from build123d import *

# Parameters (mm, degrees)
SKETCH2_R                                 = 1
SKETCH2_W                                 = 23
SKETCH2_H                                 = 12
BOSS_EXTRUDE1_DEPTH                       = 6
CUT_EXTRUDE1_REACH                        = 57.536
SKETCH3_W                                 = 10
SKETCH3_H                                 = 11
FILLET1_R                                 = 3
TAP_DRILL_FOR_M3X0_5_TAP1_D               = 2.5
TAP_DRILL_FOR_M3X0_5_TAP1_DEPTH           = 10
TAP_DRILL_FOR_M3X0_5_TAP1_TIP             = 0.751075774
TAP_DRILL_FOR_M3X0_5_TAP1_ON_FACE_2_D     = 2.5
TAP_DRILL_FOR_M3X0_5_TAP1_ON_FACE_2_DEPTH = 10
TAP_DRILL_FOR_M3X0_5_TAP1_ON_FACE_2_TIP   = 0.751075774


with BuildPart() as part:
    # Sketch2 → Boss-Extrude1 (new body)
    with BuildSketch(Plane(origin=(0, 0, 0), x_dir=(0, 0, -1), z_dir=(1, 0, 0))):
        Polygon((-20, 0), (-22.339658165, -13.268860813), (-43.5, -17), (-43.5, -34), (0, -34), (0, 0), align=None)
        with Locations(Location((-41.25, -25, 0), (0, 0, 180))):
            Circle(SKETCH2_R, mode=Mode.SUBTRACT)
        with Locations(Location((-13.75, -25, 0), (0, 0, 180))):
            Circle(SKETCH2_R, mode=Mode.SUBTRACT)
        with Locations((-27.5, -25)):
            Rectangle(SKETCH2_W, SKETCH2_H, mode=Mode.SUBTRACT)
    extrude(amount=BOSS_EXTRUDE1_DEPTH)

    # Sketch3 → Cut-Extrude1 (cut, up to next)
    with BuildSketch(Plane.ZY, mode=Mode.PRIVATE) as cut_extrude1_sk1:
        with Locations((5, -28.5)):
            Rectangle(SKETCH3_W, SKETCH3_H)
    cut_extrude1_tool1 = extrude(cut_extrude1_sk1.sketch, amount=-CUT_EXTRUDE1_REACH, mode=Mode.PRIVATE) & part.part
    add(cut_extrude1_tool1.solids().sort_by_distance((0, -28.5, 5))[0], mode=Mode.SUBTRACT)

    # Fillet1
    fillet1_edges = [part.edges().sort_by_distance(p)[0] for p in [
        (3, -34, 43.5),
        (3, -17, 43.5),
        (3, -13.268860813, 22.339658165),
        (3, -34, 10),
    ]]
    fillet(fillet1_edges, radius=FILLET1_R)

    # Tap Drill for M3x0.5 Tap1
    with Locations(Plane(origin=(3, 0, 3), x_dir=(0, 0, 1), z_dir=(0, 1, 0))):
        with Locations((0, 0), (14, 0)):
            Hole(TAP_DRILL_FOR_M3X0_5_TAP1_D / 2, depth=TAP_DRILL_FOR_M3X0_5_TAP1_DEPTH)
            with Locations((0, 0, -(TAP_DRILL_FOR_M3X0_5_TAP1_DEPTH + TAP_DRILL_FOR_M3X0_5_TAP1_TIP / 2))):  # 118° drill point
                Cone(0, TAP_DRILL_FOR_M3X0_5_TAP1_D / 2, TAP_DRILL_FOR_M3X0_5_TAP1_TIP, mode=Mode.SUBTRACT)

    # Tap Drill for M3x0.5 Tap1 on face 2
    with Locations(Plane(origin=(3, -23, 5), x_dir=(0, 0, -1), z_dir=(0, -1, 0))):
        with Locations((0, 0)):
            Hole(TAP_DRILL_FOR_M3X0_5_TAP1_ON_FACE_2_D / 2, depth=TAP_DRILL_FOR_M3X0_5_TAP1_ON_FACE_2_DEPTH)
            with Locations((0, 0, -(TAP_DRILL_FOR_M3X0_5_TAP1_ON_FACE_2_DEPTH + TAP_DRILL_FOR_M3X0_5_TAP1_ON_FACE_2_TIP / 2))):  # 118° drill point
                Cone(0, TAP_DRILL_FOR_M3X0_5_TAP1_ON_FACE_2_D / 2, TAP_DRILL_FOR_M3X0_5_TAP1_ON_FACE_2_TIP, mode=Mode.SUBTRACT)


solid = part.part
For this review, take the finished solid that the model builds, in its own axes (mm). A direction names the side the tool comes from. Round coordinates to 2 decimals unless told otherwise and drop trailing zeros. Order: outer loops, then holes, each group sorted by start corner. A loop starts at its lowest first (then second) coordinate and runs counter-clockwise, first axis right, second up. Notation, with made-up numbers: M 31,-10 L 79,-10 A18 cw 79,12 Z; hole C 29,-3.5 d4. An arc over 180 degrees is marked long. Write each question's results on one line, items separated by ' | '. Start each with the question number.
1. To check wall thickness, follow L1, parallel to Z at x = 2.5, y = -25; L2, parallel to Y at x = 1.8, z = 13.75; L3, parallel to Z at x = 3, y = -2.25. State the ranges of each line that lie inside material, in increasing order. Write a range as [from, to].
2. Add section A-A (x = 0.8). State the section outline as (y, z) points, then the cut area to 3 significant figures.
3. Draft analysis for pull direction Y (two halves, no side actions). For faces 6 (the face through (3, -25, 16)), 7 (the face through (3.04, -12.78, 22.79)), 8 (the face through (3, -34, 27)), state which applies: pulls with the +Y half, pulls with the -Y half, needs draft (parallel to the pull), parting line crosses it, or undercut.
4. Add section D-D (y = -25). State the section outline as (x, z) points.
5. Tool access review of faces 1 (the face through (3.04, -17.57, 42.78)), 2 (the face through (3, -27, 10)), 3 (the face through (3.38, -5.07, 1.81)), 4 (the face through (4.24, -17.93, 4.84)), 5 (the face through (3, -19, 28)): name each direction out of +Z, -Z, +X, -X, +Y, -Y from which nothing blocks a thin tool from reaching the whole face with its end or side.
6. Clearance check with flat-ended pins moving along their axes: pin 1 Ø1.8 at (x, y) = (3.5, -27) entering from -Z; pin 2 Ø1.2 at (y, z) = (-25, 41.25) entering from +X; pin 3 Ø1.8 at (x, z) = (3.5, 5) entering from -Y. State where each tip first meets the part, or that it passes through.
7. Add section B-B (y = -29). State the section outline as (x, z) points.
8. Add section C-C (z = 13.75). State the section outline as (x, y) points, then the cut area to 3 significant figures.
Output values:
1) L1: [10, 12.75], [14.75, 16], [39, 40.25], [42.25, 43.5] | L2: [-34, -26], [-24, 0] | L3: [0, 1.75], [4.25, 15.75], [18.25, 20.4]
2) outline: M -34,13 A3 ccw -31,10 L -23,10 L -23,0 L 0,0 L 0,20 L -11.2,21.97 A3 cw -13.63,24.41 L -16.56,41.02 A3 ccw -19.52,43.5 L -31,43.5 A3 ccw -34,40.5 Z; hole M -31,16 L -19,16 L -19,39 L -31,39 Z; hole C -25,13.75 d2; hole C -25,41.25 d2 | area: 747 mm^2
3) face 6: undercut | face 7: pulls with the +Y half | face 8: pulls with the -Y half
4) outline: M 0,10 L 6,10 L 6,12.75 L 0,12.75 Z; M 0,14.75 L 6,14.75 L 6,16 L 0,16 Z; M 0,39 L 6,39 L 6,40.25 L 0,40.25 Z; M 0,42.25 L 6,42.25 L 6,43.5 L 0,43.5 Z
5) face 1: +Z, +X, -X, +Y | face 2: -Z, +X, -X, -Y | face 3: +Y | face 4: -Y | face 5: +X, -X
6) pin 1: z = 10 | pin 2: through | pin 3: y = -23
7) outline: M 0,10 L 6,10 L 6,16 L 0,16 Z; M 0,39 L 6,39 L 6,43.5 L 0,43.5 Z
8) outline: M 0,-34 L 6,-34 L 6,-26 L 0,-26 Z; M 0,-24 L 6,-24 L 6,0 L 0,0 Z | area: 192 mm^2
